Job drawing, mm, ordinate dimensions from the low corner. One solid piece. A direction names the side the tool comes from. Give positions to 0.01 mm unless a question says otherwise; leave off trailing zeros. Loops run counter-clockwise (first coordinate to the right, second up) from the corner with the lowest first, then second, coordinate; pieces in that order, holes last.
Item 1: Saw through at B-B on x = 31.4. Give the cut face in (y, z) (1 decimal).
Item 2: Probe probe 1 along Y at (x, z) = (8, 17.25) (1 decimal); probe 2 along X at (y, z) = (8.25, 8) (1 decimal); probe 3 along X at (y, z) = (9.5, 11.5). List the from-to ranges inside material, lowest first.
Item 3: Saw through at A-A on y = 9.5. Give the cut face in (x, z), plus the area to 3 significant figures.
Item 4: Mould opens along X. For the marked faces 3, 4 and 5 say: released by +X, released by -X, zero draft, split by the parting line, or undercut.
Item 5: Saw through at C-C on z = 6.5. Give the cut face in (x, y) (1 decimal), plus the area to 3 significant figures.
Item 6: Which spindle directions (+Z, -Z, +X, -X, +Y, -Y) get a long thin tool onto all of the face, cutting with end or side? Do the marked faces 1 and 2. Say none if no direction does.
Item 7: Saw through at D-D on z = 3.5. Give the cut face in (x, y) (1 decimal), plus the area to 3 significant figures.
Item 8: Drop a flat-ended pin along its axis: P1, Ø3, axis at x = 24, y = 10.5, coming from the +Z side. Give the stop position or say it passes through.
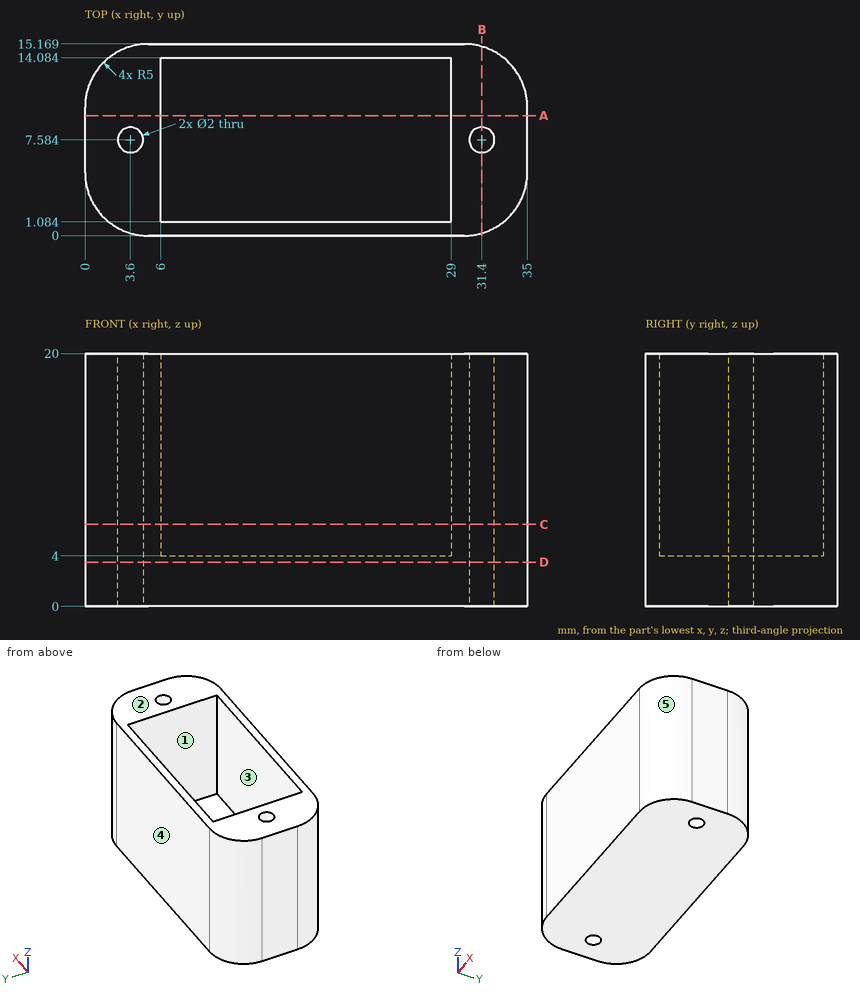
Results below:
1. outline: (0.2, 0) - (6.6, 0) - (6.6, 20) - (0.2, 20) - close; (8.6, 0) - (15, 0) - (15, 20) - (8.6, 20) - close
2. probe 1: y = 0 to 1.1, 14.1 to 15.2
2. probe 2: x = 0 to 2.9, 4.3 to 6, 29 to 30.7, 32.1 to 35
2. probe 3: x = 0 to 6, 29 to 35
3. outline: (0, 0) - (35, 0) - (35, 20) - (29, 20) - (29, 4) - (6, 4) - (6, 20) - (0, 20) - close
3. area: 332 mm2
4. face 3: undercut
4. face 4: zero draft
4. face 5: released by +X
5. outline: (0, 5) arc R5 ccw to (5, 0) - (30, 0) arc R5 ccw to (35, 5) - (35, 10.2) arc R5 ccw to (30, 15.2) - (5, 15.2) arc R5 ccw to (0, 10.2) - close; hole circle Ø2 at (3.6, 7.6); hole (6, 1.1) - (29, 1.1) - (29, 14.1) - (6, 14.1) - close; hole circle Ø2 at (31.4, 7.6)
5. area: 204 mm2
6. face 1: +Z
6. face 2: +Z, +X, -X, +Y, -Y
7. outline: (0, 5) arc R5 ccw to (5, 0) - (30, 0) arc R5 ccw to (35, 5) - (35, 10.2) arc R5 ccw to (30, 15.2) - (5, 15.2) arc R5 ccw to (0, 10.2) - close; hole circle Ø2 at (3.6, 7.6); hole circle Ø2 at (31.4, 7.6)
7. area: 503 mm2
8. P1: stops at z = 4
